Can you work these out from the model? Positions are in its coordinate system, mm. Coordinates: 2 decimals unless noted, no trailing zeros. Write each loop counter-clockwise with the first axis right and the second up, starting at its lowest first coordinate (ties: lowest second). Pieces come first, ordered by that corner, then holes.
```python
from build123d import *

# Parameters (mm, degrees)
ESQUISSE1_R                  = 40
BOSS_EXTRU_1_DEPTH           = 1
D_GAGEMENT_M21_D             = 2.6
R_P_TITION_CIRCULAIRE1_COUNT = 4


with BuildPart() as part:
    # Esquisse1 → Boss.-Extru.1 (new body)
    with BuildSketch(Plane.XY):
        Circle(ESQUISSE1_R)
    extrude(amount=BOSS_EXTRU_1_DEPTH)

    # Dégagement M21 (through all)
    with Locations(Plane(origin=(0, 0, 0), x_dir=(-1, 0, 0), z_dir=(0, 0, -1))):
        with Locations((0, 37)):
            d_gagement_m21 = Hole(D_GAGEMENT_M21_D / 2)

    # Répétition circulaire1: Dégagement M21 ×4 about axis
    r_p_tition_circulaire1_axis = Axis((0, 0, 0), (0, 0, 1))
    for i in range(1, R_P_TITION_CIRCULAIRE1_COUNT):
        add(d_gagement_m21.rotate(r_p_tition_circulaire1_axis, i * 360 / R_P_TITION_CIRCULAIRE1_COUNT), mode=Mode.SUBTRACT)


solid = part.part
```
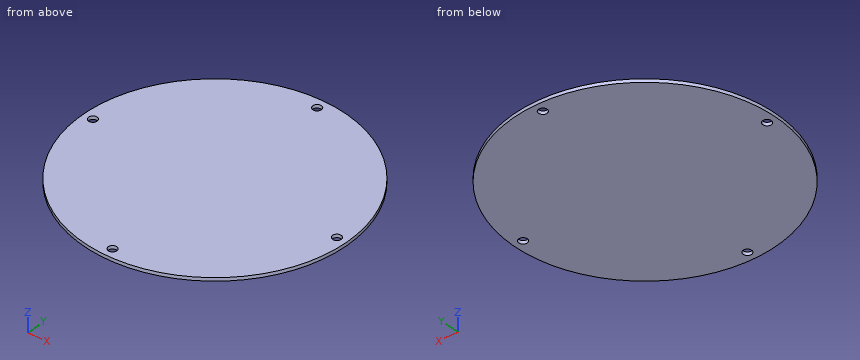
1. If we section it at D-D, the plane x = -37: List the corners of the cut face in (y, z) for me.
2. I'm going to push a flat-ended pin straight in: P1, Ø1.6, axis at x = 0, y = 37, coming from the +Z side. Where does the tip first touch, or does it pass through?
3. If we section it at A-A, the plane y = 0: List the corners of the cut face in (x, z) for me.
4. If we section it at C-C, the plane z = 0.7: List the corners of the cut face in (x, y) for me.
5. If I drill on L1, parallel to Y at x = 0, z = 0.75; L2, parallel to X at y = -37, z = 0.55, over which ranges is the centre line in solid material (lowest first)?
Answers:
1. outline: (-15.2, 0) - (-1.3, 0) - (-1.3, 1) - (-15.2, 1) - close; (1.3, 0) - (15.2, 0) - (15.2, 1) - (1.3, 1) - close
2. P1: passes through
3. outline: (-40, 0) - (-38.3, 0) - (-38.3, 1) - (-40, 1) - close; (-35.7, 0) - (35.7, 0) - (35.7, 1) - (-35.7, 1) - close; (38.3, 0) - (40, 0) - (40, 1) - (38.3, 1) - close
4. outline: circle Ø80 at (0, 0); hole circle Ø2.6 at (-37, 0); hole circle Ø2.6 at (0, -37); hole circle Ø2.6 at (0, 37); hole circle Ø2.6 at (37, 0)
5. L1: y = -40 to -38.3, -35.7 to 35.7, 38.3 to 40
5. L2: x = -15.2 to -1.3, 1.3 to 15.2
